CAD build for the part. Positions are in the model's coordinates, mm. Round coordinates to 2 decimals unless told otherwise and drop trailing zeros. Loops run counter-clockwise (first coordinate to the right, second up) from the corner with the lowest first, then second, coordinate; pieces in that order, holes last.
```python
from build123d import *

# Parameters (mm, degrees)
SKETCH_1_R          = 25
SKETCH_1_R_2        = 13
EXTRUDE_1_DEPTH     = 3
SKETCH_2_R          = 2
CUT_EXTRUDE_1_DEPTH = 3
EXTRUDE_START       = -3
EXTRUDE_2_DEPTH     = 3
SKETCH_4_W          = 100
SKETCH_4_H          = 20
EXTRUDE_3_DEPTH     = 3
EXTRUDE_4_DEPTH     = 3
SKETCH_6_R          = 2.1
CUT_EXTRUDE_2_DEPTH = 87.075548212
FILLET_1_R          = 5
FILLET_2_R          = 10


with BuildPart() as part:
    # 草图1 → 凸台-拉伸1 (new body)
    with BuildSketch(Plane(origin=(0, 0, 0), x_dir=(0, 0, -1), z_dir=(1, 0, 0))):
        Circle(SKETCH_1_R)
        Circle(SKETCH_1_R_2, mode=Mode.SUBTRACT)
    extrude(amount=EXTRUDE_1_DEPTH)

    # 草图2 → 切除-拉伸1 (cut)
    with BuildSketch(Plane(origin=(3, 0, 0), x_dir=(0, 0, -1), z_dir=(1, 0, 0))):
        with Locations((0, 17.5)):
            Circle(SKETCH_2_R)
        with Locations((17.5, 0)):
            Circle(SKETCH_2_R)
        with Locations((0, -17.5)):
            Circle(SKETCH_2_R)
        with Locations((-17.5, 0)):
            Circle(SKETCH_2_R)
    extrude(amount=-CUT_EXTRUDE_1_DEPTH, mode=Mode.SUBTRACT)

    # 草图3 → 凸台-拉伸2 (add)
    with BuildSketch(Plane(origin=(3, 0, 0), x_dir=(0, 0, -1), z_dir=(1, 0, 0)).offset(EXTRUDE_START)):
        with BuildLine():
            Line((-25, 0), (-25, 70))
            Line((-25, 70), (25, 70))
            Line((25, 70), (25, 0))
            ThreePointArc((25, 0), (0, 25), (-25, 0))
        make_face()
    extrude(amount=EXTRUDE_2_DEPTH)

    # 草图4 → 凸台-拉伸3 (add)
    with BuildSketch(Plane(origin=(3, 0, 0), x_dir=(0, 0, -1), z_dir=(1, 0, 0))):
        with Locations((0, 60)):
            Rectangle(SKETCH_4_W, SKETCH_4_H)
    extrude(amount=-EXTRUDE_3_DEPTH)

    # 草图5 → 凸台-拉伸4 (add)
    with BuildSketch(Plane(origin=(3, 0, 0), x_dir=(0, 0, -1), z_dir=(1, 0, 0)).offset(EXTRUDE_START)):
        with BuildLine():
            Line((-22.785945694, -10.285945694), (-50, 50))
            Line((-50, 50), (-25, 50))
            Line((-25, 50), (-25, 0))
            ThreePointArc((-25, 0), (-24.440219336, -5.260767893), (-22.785945694, -10.285945694))
        make_face()
        with BuildLine():
            Line((22.785945694, -10.285945694), (50, 50))
            Line((50, 50), (25, 50))
            Line((25, 50), (25, 0))
            ThreePointArc((25, 0), (24.440219336, -5.260767893), (22.785945694, -10.285945694))
        make_face()
    extrude(amount=EXTRUDE_4_DEPTH)

    # 草图6 → 切除-拉伸2 (cut, through all)
    with BuildSketch(Plane(origin=(3, 0, 0), x_dir=(0, 0, -1), z_dir=(1, 0, 0))):
        with Locations((-40, 60)):
            Circle(SKETCH_6_R)
        with Locations((0, 60)):
            Circle(SKETCH_6_R)
        with Locations((40, 60)):
            Circle(SKETCH_6_R)
    extrude(amount=-CUT_EXTRUDE_2_DEPTH, mode=Mode.SUBTRACT)

    # 圆角1
    fillet_1_edges = [part.edges().sort_by_distance(p)[0] for p in [
        (1.5, 70, 50),
        (1.5, 70, -50),
    ]]
    fillet(fillet_1_edges, radius=FILLET_1_R)

    # 圆角2
    fillet_2_edges = [part.edges().sort_by_distance(p)[0] for p in [
        (1.5, 50, 50),
        (1.5, 50, -50),
    ]]
    fillet(fillet_2_edges, radius=FILLET_2_R)


solid = part.part
```
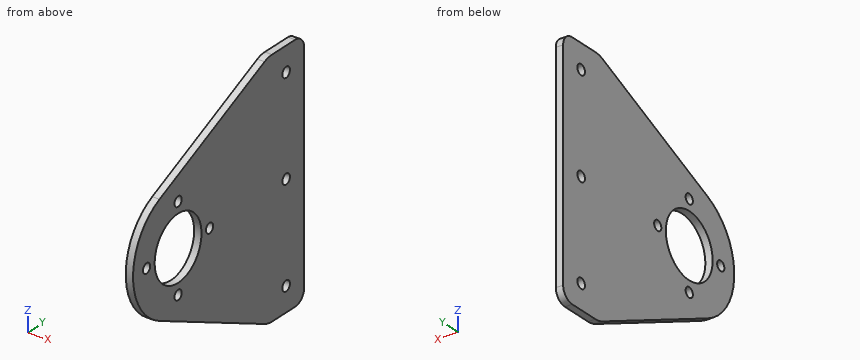
Item 1: Flat gauge pin, fed straight in: P1, Ø1.5, axis at x = 0.5, y = -1.5, coming from the -Z side. Where does the tip first touch, or does it go through?
Answers follow:
P1: stops at z = -27.09
Item 2: Cut at C-C, the plane y = 60. Give the cut face in (x, z), plus the area to 3 significant figures.
Answers follow:
outline: (0, -50) - (3, -50) - (3, -42.1) - (0, -42.1) - close; (0, -37.9) - (3, -37.9) - (3, -2.1) - (0, -2.1) - close; (0, 2.1) - (3, 2.1) - (3, 37.9) - (0, 37.9) - close; (0, 42.1) - (3, 42.1) - (3, 50) - (0, 50) - close
area: 262 mm2
Item 3: Cut at B-B, the plane x = 0.5. State how many separate pieces and enclosed holes the cut face has, plus the area to 3 significant figures.
Answers follow:
separate pieces: 1
enclosed holes: 8
area: 6,240 mm2
Item 4: Probe line 1 (Y direction, x = 1.95, z = 0); line 2 (Z direction, x = 1.5, y = 61.5); line 3 (Y direction, x = 2.65, z = -8.5). List the from-to ranges inside material, lowest first.
Answers follow:
line 1: y = -25 to -19.5, -15.5 to -13, 13 to 15.5, 19.5 to 57.9, 62.1 to 70
line 2: z = -50 to -41.47, -38.53 to -1.47, 1.47 to 38.53, 41.47 to 50
line 3: y = -23.51 to -9.84, 9.84 to 70
Item 5: Cut at D-D, the plane y = -17.5. Give the cut face in (x, z), plus the area to 3 significant figures.
Answers follow:
outline: (0, -17.85) - (3, -17.85) - (3, -2) - (0, -2) - close; (0, 2) - (3, 2) - (3, 17.85) - (0, 17.85) - close
area: 95.1 mm2
Item 6: Cut at A-A, the plane z = 0. Give the cut face in (x, y).
Answers follow:
outline: (0, -25) - (3, -25) - (3, -19.5) - (0, -19.5) - close; (0, -15.5) - (3, -15.5) - (3, -13) - (0, -13) - close; (0, 13) - (3, 13) - (3, 15.5) - (0, 15.5) - close; (0, 19.5) - (3, 19.5) - (3, 57.9) - (0, 57.9) - close; (0, 62.1) - (3, 62.1) - (3, 70) - (0, 70) - close
